from build123d import *

# Parameters (mm, degrees)
SKETCH1_W           = 76
SKETCH1_H           = 10
BOSS_EXTRUDE1_DEPTH = 4
SKETCH2_R           = 1.5
CUT_EXTRUDE1_DEPTH  = 4
CUT_EXTRUDE2_DEPTH  = 10
FILLET1_R           = 1


with BuildPart() as part:
    # Sketch1 → Boss-Extrude1 (new body)
    with BuildSketch(Plane(origin=(0, 0, 0), x_dir=(1, 0, 0), z_dir=(0, 1, 0))):
        Rectangle(SKETCH1_W, SKETCH1_H)
    extrude(amount=BOSS_EXTRUDE1_DEPTH)

    # Sketch2 → Cut-Extrude1 (cut)
    with BuildSketch(Plane(origin=(0, 4, 0), x_dir=(1, 0, 0), z_dir=(0, 1, 0))):
        with Locations(Location((-34, 0, 0), (0, 0, 270))):
            Circle(SKETCH2_R)
        with Locations(Location((34, 0, 0), (0, 0, 270))):
            Circle(SKETCH2_R)
    extrude(amount=-CUT_EXTRUDE1_DEPTH, mode=Mode.SUBTRACT)

    # Sketch3 → Cut-Extrude2 (cut)
    with BuildSketch(Plane(origin=(0, 4, 0), x_dir=(1, 0, 0), z_dir=(0, 1, 0))):
        Polygon((-28, 5), (-23.669872981, 2.5), (23.669872981, 2.5), (28, 5), align=None)
        Polygon((-28, -5), (-23.669872981, -2.5), (23.669872981, -2.5), (28, -5), align=None)
    extrude(amount=-CUT_EXTRUDE2_DEPTH, mode=Mode.SUBTRACT)

    # Fillet1
    fillet1_edges = [part.edges().sort_by_distance(p)[0] for p in [
        (-38, 4, 0),
        (-33, 4, 5),
        (33, 0, 5),
        (-33, 0, -5),
        (25.834936491, 0, 3.75),
        (0, 0, 2.5),
        (-25.834936491, 0, 3.75),
        (-25.834936491, 0, -3.75),
        (0, 0, -2.5),
        (25.834936491, 0, -3.75),
        (-33, 4, -5),
        (33, 4, 5),
        (-28, 2, -5),
        (28, 2, -5),
        (23.669872981, 2, -2.5),
        (-23.669872981, 2, -2.5),
        (-25.834936491, 4, -3.75),
        (0, 4, -2.5),
        (25.834936491, 4, -3.75),
        (28, 2, 5),
        (-28, 2, 5),
        (-23.669872981, 2, 2.5),
        (23.669872981, 2, 2.5),
        (25.834936491, 4, 3.75),
        (0, 4, 2.5),
        (-25.834936491, 4, 3.75),
        (38, 4, 0),
        (-33, 0, 5),
        (-38, 0, 0),
        (33, 0, -5),
        (38, 0, 0),
        (38, 2, 5),
        (-38, 2, 5),
        (-38, 2, -5),
        (38, 2, -5),
        (33, 4, -5),
    ]]
    fillet(fillet1_edges, radius=FILLET1_R)


solid = part.part
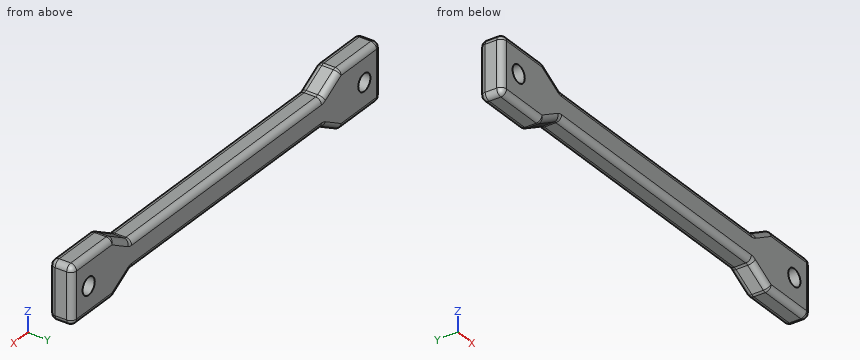
The listing builds one solid part. Answer for the finished solid, in the listing's coordinates (mm). Round coordinates to 2 decimals unless told otherwise and drop trailing zeros. Loops run counter-clockwise (first coordinate to the right, second up) from the corner with the lowest first, then second, coordinate; pieces in that order, holes last. Notation, with made-up numbers: M -12,62 L -3,62 A36 cw -3,99 Z; hole C 55.25,-35 d5. An arc over 180 degrees is marked long. Write each question's results on one line, items separated by ' | '. Start each with the question number.
1) Find section D-D on x = 29. Write down the section's boundary in (y, z).
2) Straight lines are drawn through the part: probe 1 along X at (y, z) = (1.9, 0); probe 2 along X at (y, z) = (2.15, -0.5); probe 3 along X at (y, z) = (0.3, -3.5). For each, find the intervals that lie inside material, in ascending order.
3) Find section B-B on z = 0. Write down the section's boundary in (x, y), plus the area to 3 significant figures.
4) Each of these flat-tipped pins is pushed along its axis until it touches: pin 1 (1.8 mm diameter, centred on x = -34, z = 0, fed in from -Y); pin 2 (0.6 mm diameter, centred on x = -1.5, y = 2, fed in from -Z); pin 3 (3.5 mm diameter, centred on x = 34, z = 0, fed in from -Y); pin 4 (1 mm diameter, centred on x = -1, y = 2, fed in from +Z). Where does it stop, or does it pass through?
5) Find section A-A on x = -34. Write down the section's boundary in (y, z), plus the area to 3 significant figures.
6) Find section C-C on y = 1.9. Write down the section's boundary in (x, z).
Final values:
1) outline: M 0,-4 A1 ccw 1,-5 L 3,-5 A1 ccw 4,-4 L 4,4 A1 ccw 3,5 L 1,5 A1 ccw 0,4 Z
2) probe 1: -38 to -35.5, -32.5 to 32.5, 35.5 to 38 | probe 2: -38 to -35.41, -32.59 to 32.59, 35.41 to 38 | probe 3: -37.71 to -25.97, 25.97 to 37.71
3) outline: M -38,1 A1 ccw -37,0 L -35.5,0 L -35.5,4 L -37,4 A1 ccw -38,3 Z; M -32.5,0 L 32.5,0 L 32.5,4 L -32.5,4 Z; M 35.5,0 L 37,0 A1 ccw 38,1 L 38,3 A1 ccw 37,4 L 35.5,4 Z | area: 279 mm²
4) pin 1: through | pin 2: z = -2.5 | pin 3: y = 0 | pin 4: z = 2.5
5) outline: M 0,-4 A1 ccw 1,-5 L 3,-5 A1 ccw 4,-4 L 4,-1.5 L 0,-1.5 Z; M 0,1.5 L 4,1.5 L 4,4 A1 ccw 3,5 L 1,5 A1 ccw 0,4 Z | area: 27.1 mm²
6) outline: M -38,-4 A1 ccw -37,-5 L -28.27,-5 A1 ccw -27.77,-4.87 L -23.9,-2.63 A1 cw -23.4,-2.5 L 23.4,-2.5 A1 cw 23.9,-2.63 L 27.77,-4.87 A1 ccw 28.27,-5 L 37,-5 A1 ccw 38,-4 L 38,4 A1 ccw 37,5 L 28.27,5 A1 ccw 27.77,4.87 L 23.9,2.63 A1 cw 23.4,2.5 L -23.4,2.5 A1 cw -23.9,2.63 L -27.77,4.87 A1 ccw -28.27,5 L -37,5 A1 ccw -38,4 Z; hole C -34,0 d3; hole C 34,0 d3
